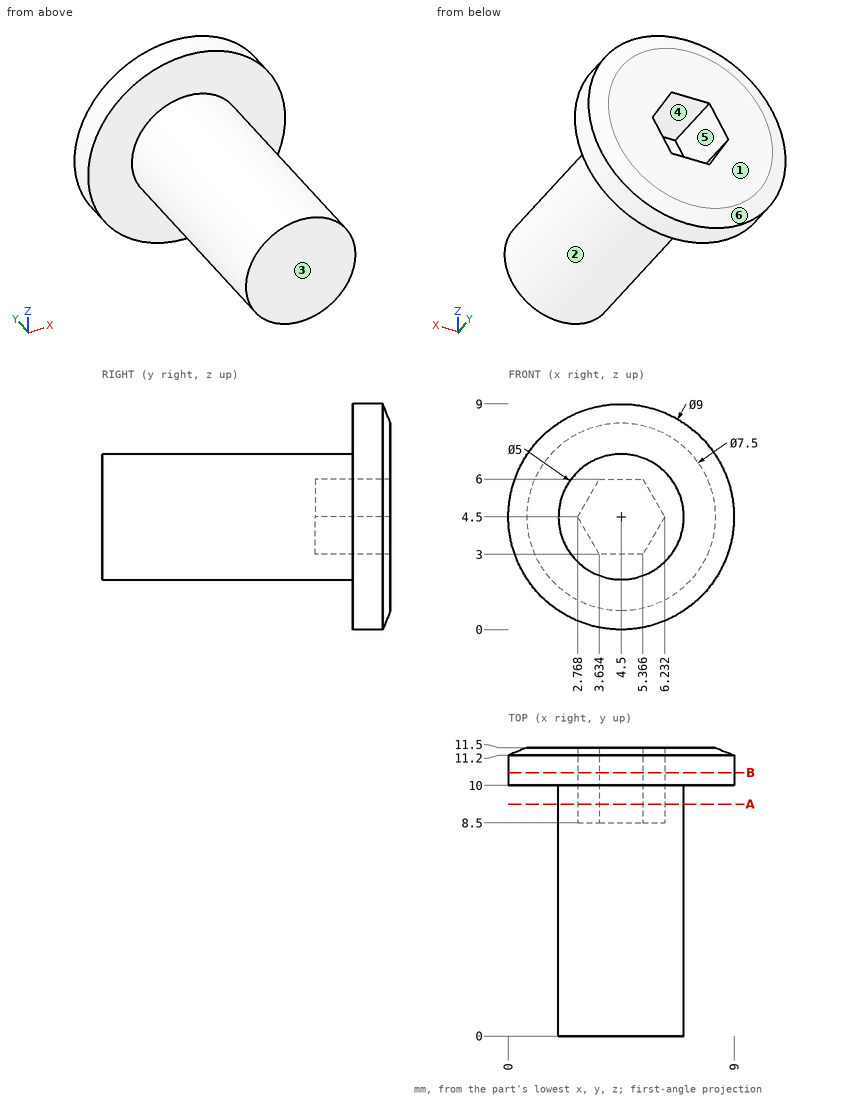
Job drawing, mm, ordinate dimensions from the low corner. One solid piece. A direction names the side the tool comes from. Give positions to 0.01 mm unless a question says otherwise; leave off trailing zeros. Loops run counter-clockwise (first coordinate to the right, second up) from the corner with the lowest first, then second, coordinate; pieces in that order, holes last. Notation, with made-up numbers: (54, -21) - (79, -21) arc R25 ccw to (79, 6) - close; hole circle Ø2 at (62.5, 12.5). An arc over 180 degrees is marked (long way). Use one line per item in the form item = value.
(1) 3-axis set-ups, long thin cutter, end or side, ignore diameter. For the marked faces 1 and 2: which of +Z, -Z, +X, -X, +Y, -Y reach the whole face in a straight line?
Determined:
face_1 = +Z, -Z, +X, -X, +Y
face_2 = -Y
(2) Cut at B-B (y = 10.5). Give the cut face in (x, z), then the cut area to 3 significant figures.
Determined:
outline = circle Ø9 at (4.5, 4.5); hole (2.77, 4.5) - (3.63, 3) - (5.37, 3) - (6.23, 4.5) - (5.37, 6) - (3.63, 6) - close
area = 55.8 mm^2
(3) Drop flat-ended pins along their axis: P1, Ø1, axis at x = 4.5, y = 1, coming from the +Z side; P2, Ø4, axis at y = 5, z = 4, coming from the -X side; P3, Ø3.5, axis at x = 5, z = 5, coming from the +Y side; P4, Ø3, axis at x = 1.5, y = 6.5, coming from the -Z side. Give the stop position or say it passes through.
Determined:
P1 = 7
P2 = 2
P3 = 11.5
P4 = 2.5
(4) Cut at A-A (y = 9.25). Give the cut face in (x, z).
Determined:
outline = circle Ø5 at (4.5, 4.5); hole (2.77, 4.5) - (3.63, 3) - (5.37, 3) - (6.23, 4.5) - (5.37, 6) - (3.63, 6) - close
(5) Drill centre lines: L1, parallel to Z at x = 5, y = 11; L2, parallel to Z at x = 6.5, y = 2.75; L3, parallel to Y at x = 3.25, z = 8. Where is each one in solid material? Low to high.
Determined:
L1 = 0.03 to 3, 6 to 8.97
L2 = 3 to 6
L3 = 10 to 11.5
(6) Pull direction X, two halves, no side cores. Call the marked faces 3, 4, 5 and 6: pulls with the +X half, pulls with the -X half, needs draft (parallel to the pull), parting line crosses it, or undercut.
Determined:
face_3 = needs draft
face_4 = undercut
face_5 = undercut
face_6 = parting line crosses it
